Can you work these out from the drawing? Everything is in mm from the part's minimum corner. A direction names the side the tool comes from. Give positions to 0.01 mm unless a question says otherwise; leave off trailing zeros. Order: outer loops, then holes, each group sorted by start corner. A loop starts at its lowest first (then second) coordinate and runs counter-clockwise, first axis right, second up. Notation, with made-up numbers: (76, 4.5) - (127, 4.5) arc R27 ccw to (127, 30.5) - close; hole circle Ø3 at (26.5, -12). An arc over 180 degrees is marked (long way). Answer as a JSON object with one key per item and string values.
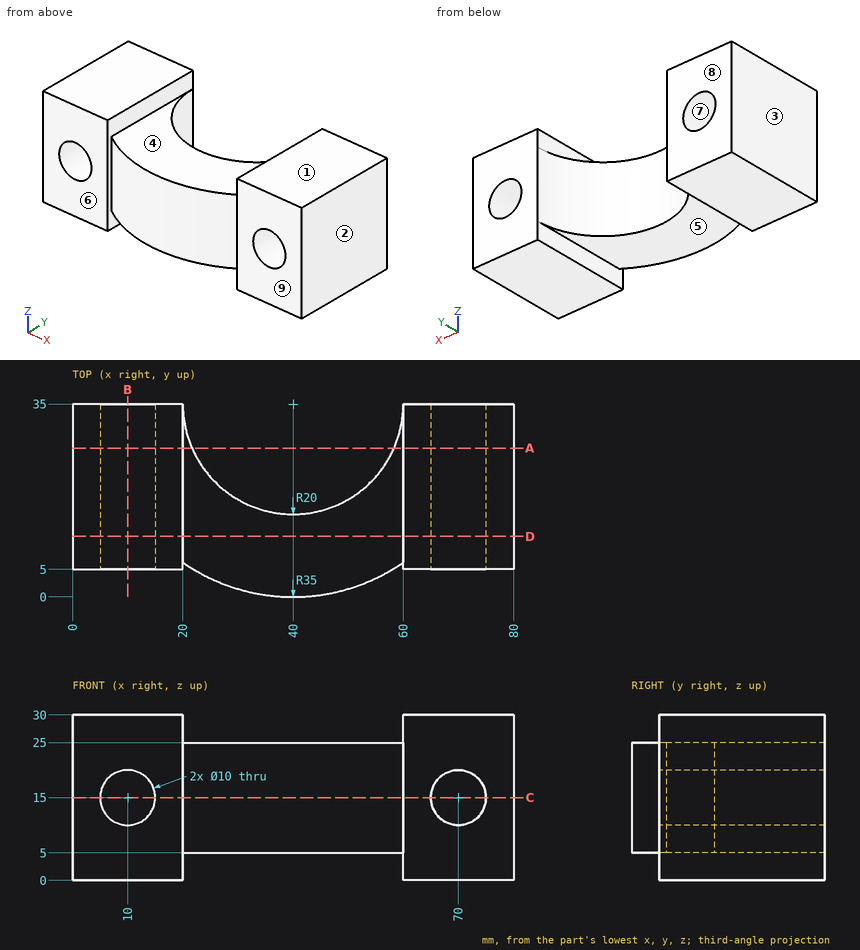
Q1. If we section it at B-B, the plane x = 10: Please give me the cut outline in (y, z), then the cut area to 3 significant figures.
Recorded:
{"outline": "(5, 0) - (35, 0) - (35, 10) - (5, 10) - close; (5, 20) - (35, 20) - (35, 30) - (5, 30) - close", "area": "600 mm^2"}
Q2. I need wall thicknesses on L1, parallel to Z at x = 10, y = 28; L2, parallel to X at y = 9.5, z = 17.25; L3, parallel to X at y = 17.75, z = 15. Which ranges of each line are inside material? Lowest first, please.
Recorded:
{"L1": "z = 0 to 10, 20 to 30", "L2": "x = 0 to 5.53, 14.47 to 65.53, 74.47 to 80", "L3": "x = 0 to 5, 15 to 29.88, 50.12 to 65, 75 to 80"}
Q3. We'd pull the mould along X, two halves only. Please class the marked faces 1, 2, 3 and 4: released by +X, released by -X, zero draft, split by the parting line, or undercut.
Recorded:
{"face 1": "zero draft", "face 2": "released by +X", "face 3": "released by -X", "face 4": "undercut"}
Q4. If we section it at A-A, the plane y = 27: Please give me the cut outline in (x, z), then the cut area to 3 significant figures.
Recorded:
{"outline": "(0, 0) - (20, 0) - (20, 5) - (21.67, 5) - (21.67, 25) - (20, 25) - (20, 30) - (0, 30) - close; (58.33, 5) - (60, 5) - (60, 0) - (80, 0) - (80, 30) - (60, 30) - (60, 25) - (58.33, 25) - close; hole circle Ø10 at (10, 15); hole circle Ø10 at (70, 15)", "area": "1,110 mm^2"}
Q5. Which directions (+Z, -Z, +X, -X, +Y, -Y) give clear straight access to the entire face, cutting with the end or side of a thin tool? Please do the marked faces 5, 6, 7, 8 and 9.
Recorded:
{"face 5": "-Z, +Y, -Y", "face 6": "+Z, -Z, -X, -Y", "face 7": "+Y, -Y", "face 8": "+Z, -Z, +X, -X, +Y", "face 9": "+Z, -Z, +X, -Y"}
Q6. If we section it at D-D, the plane y = 11: Please give me the cut outline in (x, z), then the cut area to 3 significant figures.
Recorded:
{"outline": "(0, 0) - (20, 0) - (20, 5) - (60, 5) - (60, 0) - (80, 0) - (80, 30) - (60, 30) - (60, 25) - (20, 25) - (20, 30) - (0, 30) - close; hole circle Ø10 at (10, 15); hole circle Ø10 at (70, 15)", "area": "1,840 mm^2"}
Q7. I'm going to push flat-ended pins straight in: pin 1 Ø4 at (y, z) = (15.5, 5) entering from -X; pin 2 Ø3 at (x, z) = (31.5, 16) entering from -Y; pin 3 Ø5 at (x, z) = (38.5, 21) entering from +Y; pin 4 Ø11.5 at (x, z) = (10, 15) entering from -Y. Where does each tip first touch, or does it pass through?
Recorded:
{"pin 1": "stops at x = 0", "pin 2": "stops at y = 0.71", "pin 3": "stops at y = 15.4", "pin 4": "stops at y = 5"}
Q8. If we section it at C-C, the plane z = 15: Please give me the cut outline in (x, y), then the cut area to 3 significant figures.
Recorded:
{"outline": "(0, 5) - (5, 5) - (5, 35) - (0, 35) - close; (15, 5) - (20, 5) - (20, 6.28) arc R35 ccw to (60, 6.28) - (60, 5) - (65, 5) - (65, 35) - (60, 35) arc R20 cw to (20, 35) - (15, 35) - close; (75, 5) - (80, 5) - (80, 35) - (75, 35) - close", "area": "1,290 mm^2"}
